from build123d import *

# Parameters (mm, degrees)
SKETCH40_W          = 220
SKETCH40_H          = 140
BOSS_EXTRUDE7_DEPTH = 3.175
SKETCH41_W          = 20
SKETCH41_H          = 3.175
SKETCH41_W_2        = 3.175
SKETCH41_H_2        = 20
CUT_EXTRUDE21_DEPTH = 3.175
SKETCH53_W          = 60.8
SKETCH53_H          = 59.3
CUT_EXTRUDE26_DEPTH = 3.175


with BuildPart() as part:
    # Sketch40 → Boss-Extrude7 (new body)
    with BuildSketch(Plane(origin=(0, 0, 0), x_dir=(1, 0, 0), z_dir=(0, 1, 0))):
        with Locations((-4.2e-06, -668.101928689)):
            Rectangle(SKETCH40_W, SKETCH40_H)
    extrude(amount=BOSS_EXTRUDE7_DEPTH)

    # Sketch41 → Cut-Extrude21 (cut)
    with BuildSketch(Plane(origin=(0, 3.175, 0), x_dir=(1, 0, 0), z_dir=(0, 1, 0))):
        with Locations((59.9999958, -736.514428689)):
            Rectangle(SKETCH41_W, SKETCH41_H)
        Polygon((109.9999958, -738.101928689), (89.9999958, -738.101928689), (89.9999958, -734.926928689), (106.8249958, -734.926928689), (106.8249958, -718.101928689), (109.9999958, -718.101928689), align=None)
        with Locations((19.9999958, -736.514428689)):
            Rectangle(SKETCH41_W, SKETCH41_H)
        with Locations((-20.0000042, -736.514428689)):
            Rectangle(SKETCH41_W, SKETCH41_H)
        with Locations((-60.0000042, -736.514428689)):
            Rectangle(SKETCH41_W, SKETCH41_H)
        Polygon((-90.0000042, -738.101928689), (-90.0000042, -734.926928689), (-106.8250042, -734.926928689), (-106.8250042, -718.101928689), (-110.0000042, -718.101928689), (-110.0000042, -738.101928689), align=None)
        with Locations((59.9999958, -599.689428689)):
            Rectangle(SKETCH41_W, SKETCH41_H)
        Polygon((109.9999958, -598.101928689), (89.9999958, -598.101928689), (89.9999958, -601.276928689), (106.8249958, -601.276928689), (106.8249958, -618.101928689), (109.9999958, -618.101928689), align=None)
        with Locations((19.9999958, -599.689428689)):
            Rectangle(SKETCH41_W, SKETCH41_H)
        with Locations((-20.0000042, -599.689428689)):
            Rectangle(SKETCH41_W, SKETCH41_H)
        with Locations((-60.0000042, -599.689428689)):
            Rectangle(SKETCH41_W, SKETCH41_H)
        Polygon((-90.0000042, -598.101928689), (-90.0000042, -601.276928689), (-106.8250042, -601.276928689), (-106.8250042, -618.101928689), (-110.0000042, -618.101928689), (-110.0000042, -598.101928689), align=None)
        with Locations((108.4124958, -648.101928689)):
            Rectangle(SKETCH41_W_2, SKETCH41_H_2)
        with Locations((108.4124958, -688.101928689)):
            Rectangle(SKETCH41_W_2, SKETCH41_H_2)
        with Locations((-108.4125042, -648.101928689)):
            Rectangle(SKETCH41_W_2, SKETCH41_H_2)
        with Locations((-108.4125042, -688.101928689)):
            Rectangle(SKETCH41_W_2, SKETCH41_H_2)
    extrude(amount=-CUT_EXTRUDE21_DEPTH, mode=Mode.SUBTRACT)

    # Sketch53 → Cut-Extrude26 (cut)
    with BuildSketch(Plane(origin=(0, 3.175, 0), x_dir=(1, 0, 0), z_dir=(0, 1, 0))):
        with Locations((-0.4, -655.251928689)):
            Rectangle(SKETCH53_W, SKETCH53_H)
    extrude(amount=-CUT_EXTRUDE26_DEPTH, mode=Mode.SUBTRACT)


solid = part.part
Read the model definition and answer for the solid it produces. Units are mm, in the model's axes. Give positions to 0.01 mm unless a question says otherwise; leave off trailing zeros. Loops run counter-clockwise (first coordinate to the right, second up) from the corner with the lowest first, then second, coordinate; pieces in that order, holes last. Notation, with made-up numbers: (52, 86.25) - (110, 86.25) arc R26 cw to (110, 121.25) - close; hole circle Ø4 at (31.5, 56.5). An arc over 180 degrees is marked (long way). Answer as CSV lines item,"result". Start each with the question number.
1) Straight lines are drawn through the part: L1, parallel to Z at x = 28.5, y = 0.8; L2, parallel to X at y = 2.5, z = 663; L3, parallel to X at y = 2.75, z = 684 (3 decimals). For each, find the intervals that lie inside material, in ascending order. Write a range as from..to.
2) Find section A-A (z = 634). Write down the section's boundary in (x, y) (3 decimals), then the cut area to 3 significant figures.
3) Each of these flat-tipped pins is pushed along its axis until it touches: pin 1 Ø1.6 at (y, z) = (2, 599.5) entering from +X; pin 2 Ø1.6 at (x, y) = (-108, 1.5) entering from +Z; pin 3 Ø1 at (y, z) = (2, 599) entering from -X. Where does it stop, or does it pass through?
4) Find section C-C (x = 57.5). Write down the section's boundary in (y, z) (3 decimals).
5) Find section B-B (x = -19). Write down the section's boundary in (y, z) (3 decimals), then the cut area to 3 significant figures.
Findings below:
1,L1,"601.28..625.6, 684.9..734.93"
1,L2,"-110..-30.8, 30..110"
1,L3,"-106.825..-30.8, 30..106.825"
2,outline,"(-110, 0) - (-30.8, 0) - (-30.8, 3.175) - (-110, 3.175) - close; (30, 0) - (110, 0) - (110, 3.175) - (30, 3.175) - close"
2,area,"505 mm^2"
3,pin 1,"x = 90"
3,pin 2,"z = 718.1"
3,pin 3,"x = -90"
4,outline,"(0, 601.277) - (3.175, 601.277) - (3.175, 734.927) - (0, 734.927) - close"
5,outline,"(0, 601.277) - (3.175, 601.277) - (3.175, 625.602) - (0, 625.602) - close; (0, 684.902) - (3.175, 684.902) - (3.175, 734.927) - (0, 734.927) - close"
5,area,"236 mm^2"
